from build123d import *

# Parameters (mm, degrees)
SKETCH1_W           = 27.94
SKETCH1_H           = 53.34
BOSS_EXTRUDE1_DEPTH = 4.60375
SHELL1_T            = -2.54
SKETCH2_W           = 10.795
SKETCH2_H           = 1.5875
CUT_EXTRUDE1_DEPTH  = 2.54
SKETCH3_W           = 25.4
SKETCH3_H           = 50.8
CUT_EXTRUDE2_DEPTH  = 1.5875


with BuildPart() as part:
    # Sketch1 → Boss-Extrude1 (new, symmetric)
    with BuildSketch(Plane.XY):
        Rectangle(SKETCH1_W, SKETCH1_H)
    extrude(amount=BOSS_EXTRUDE1_DEPTH, both=True)

    # Shell1
    shell1_openings = [part.faces().sort_by_distance(p)[0] for p in [
        (0, 0, 4.60375),
    ]]
    offset(amount=SHELL1_T, openings=shell1_openings, kind=Kind.INTERSECTION)

    # Sketch2 → Cut-Extrude1 (cut)
    with BuildSketch(Plane(origin=(0, 26.67, 0), x_dir=(1, 0, 0), z_dir=(0, 1, 0))):
        with Locations((0, -3.81)):
            Rectangle(SKETCH2_W, SKETCH2_H)
    extrude(amount=-CUT_EXTRUDE1_DEPTH, mode=Mode.SUBTRACT)

    # Sketch3 → Cut-Extrude2 (cut)
    with BuildSketch(Plane.XY.offset(4.60375)):
        Rectangle(SKETCH3_W, SKETCH3_H)
    extrude(amount=-CUT_EXTRUDE2_DEPTH, mode=Mode.SUBTRACT)


solid = part.part
For this review, take the finished solid that the model builds, in its own axes (mm). A direction names the side the tool comes from. Coordinates: 2 decimals unless noted, no trailing zeros. Loops run counter-clockwise (first coordinate to the right, second up) from the corner with the lowest first, then second, coordinate; pieces in that order, holes last. Notation, with made-up numbers: (39.5, -11.5) - (80.5, -11.5) arc R31 ccw to (80.5, 24.5) - close; hole circle Ø10 at (32.25, 33). An arc over 180 degrees is marked (long way). Use a Markdown table: item, result. Add a question column.
Item 1: Insertion check: pin 1 Ø12.5 at (x, y) = (2.5, 3) entering from +Z; pin 2 Ø0.5 at (x, z) = (-2, 4) entering from +Y; pin 3 Ø4 at (x, y) = (10, -12.5) entering from +Z. Each pin has a flat end and moves straight along its axis. Give the tip position at first contact, or say it passes through.
Item 2: We need section B-B (x = -12). Give the boundary of the cut face in (y, z), and give its area (3 significant figures).
Item 3: We need section A-A (z = 0.5). Give the boundary of the cut face in (x, y), and give its area (3 significant figures).
Item 4: For line 1 (X direction, y = 22.5, z = 2); line 2 (Y direction, x = 6.25, z = 0.5); line 3 (Y direction, x = -9.5, z = 3.25), list the stretches that pass through material, from the lowest coordinate up.
Item 5: Mouldability with a two-part tool opening along X and no side actions: class faces 1 (the face through (-9, 25.4, 4)), 2 (the face through (0, -26.67, 0)), 3 (the face through (-13.97, 0, 0)) as pulls with the +X half, pulls with the -X half, needs draft (parallel to the pull), parting line crosses it, or undercut.
Item 6: We need section C-C (y = -19). Give the boundary of the cut face in (x, z), and give its area (3 significant figures).
Item 7: We need section D-D (x = 0). Give the boundary of the cut face in (y, z), and give its area (3 significant figures).
Item 8: Tool access review of faces 4 (the face through (-5.398, 26, 4)), 5 (the face through (0, 0, -4.604)), 6 (the face through (9, 25.4, 4)): name each direction out of +Z, -Z, +X, -X, +Y, -Y from which nothing blocks a thin tool from reaching the whole face with its end or side.
Results list:
| question | item | result |
|---|---|---|
| 1 | pin 1 | stops at z = -2.06 |
| 1 | pin 2 | stops at y = -25.4 |
| 1 | pin 3 | stops at z = 3.02 |
| 2 | outline | (-26.67, -4.6) - (26.67, -4.6) - (26.67, 4.6) - (25.4, 4.6) - (25.4, 3.02) - (-25.4, 3.02) - (-25.4, 4.6) - (-26.67, 4.6) - close |
| 2 | area | 410 mm^2 |
| 3 | outline | (-13.97, -26.67) - (13.97, -26.67) - (13.97, 26.67) - (-13.97, 26.67) - close; hole (-11.43, -24.13) - (11.43, -24.13) - (11.43, 24.13) - (-11.43, 24.13) - close |
| 3 | area | 387 mm^2 |
| 4 | line 1 | x = -13.97 to -11.43, 11.43 to 13.97 |
| 4 | line 2 | y = -26.67 to -24.13, 24.13 to 26.67 |
| 4 | line 3 | y = -26.67 to -25.4, 25.4 to 26.67 |
| 5 | face 1 | undercut |
| 5 | face 2 | needs draft |
| 5 | face 3 | pulls with the -X half |
| 6 | outline | (-13.97, -4.6) - (13.97, -4.6) - (13.97, 4.6) - (12.7, 4.6) - (12.7, 3.02) - (11.43, 3.02) - (11.43, -2.06) - (-11.43, -2.06) - (-11.43, 3.02) - (-12.7, 3.02) - (-12.7, 4.6) - (-13.97, 4.6) - close |
| 6 | area | 101 mm^2 |
| 7 | outline | (-26.67, -4.6) - (26.67, -4.6) - (26.67, 3.02) - (24.13, 3.02) - (24.13, -2.06) - (-24.13, -2.06) - (-24.13, 3.02) - (-25.4, 3.02) - (-25.4, 4.6) - (-26.67, 4.6) - close |
| 7 | area | 163 mm^2 |
| 8 | face 4 | +Z, +Y |
| 8 | face 5 | -Z, +X, -X, +Y, -Y |
| 8 | face 6 | +Z |
